Autodesk Inventor part; units mm, degrees
ref_plane "YZ Plane" through (0, 0, 0) normal (1, 0, 0) x (0, 1, 0)
ref_plane "XZ Plane" through (0, 0, 0) normal (0, 1, 0) x (-1, 0, 0)
ref_plane "XY Plane" through (0, 0, 0) normal (0, 0, 1) x (1, 0, 0)
ref_plane "Arbeitsebene1" through (107, -8, 0) normal (-1, 0, 0) x (0, 0, 1)
sketch "Skizze1" plane through (107, -8, 0) normal (-1, 0, 0) x (0, 0, 1)
  line L0 (-4.1, -2) -> (-4.1, -37.1)
  line L1 (0, -2) -> (-4.1, -2)
  line L2 (0, -37.1) -> (0, -2)
  line L3 (0, -37.1) -> (-4.1, -37.1)
  line L4 (0, -37.1) -> (10.7454, -47.8454)
  line L5 (0, -37.1) -> (15.1963, -37.1) construction
  line L6 (10.7454, -47.8454) -> (10.7454, -97.8454)
  line L7 (10.7454, -97.8454) -> (-49.2546, -97.8454)
  line L8 (-49.2546, -97.8454) -> (-49.2546, -102.8454)
  line L9 (-49.2546, -102.8454) -> (15.7454, -102.8454)
  line L10 (15.7454, -102.8454) -> (15.7454, -45.7743)
  line L11 (15.7454, -45.7743) -> (5, -35.0289)
  line L12 (5, -35.0289) -> (5, -2)
  line L13 (5, -2) -> (0, -2)
  line L14 (0, -37.1) -> (0, -2)
  point P0 (0, 8)
  dimension "d0" = 45
  dimension "d1" = 5
  dimension "d2" = 5
  dimension "d3" = 5
  dimension "d4" = 5
  dimension "d5" = 60
  dimension "d6" = 50
extrude "Extrusion1" add sketch "Skizze1" against normal blind 5 contours L13 L12 L11 L10 L9 L8 L7 L6 L4 L2
sketch "Skizze2" plane through (107, -43.0289, 5) normal (0, 0, 1) x (1, 0, 0)
  line L0 (0, 0) -> (0, 33.0289)
  line L1 (0, 0) -> (5, 0)
  line L2 (5, 33.0289) -> (5, 0)
  line L3 (0, 33.0289) -> (5, 33.0289)
  circle A0 centre (2.5, 27.9533) radius 0.9
  circle A1 centre (2.5, 6.9011) radius 0.9
  point P0 (-107, 43.0289)
  dimension "d9" = 1.8
  dimension "d10" = 1.8
extrude "Extrusion2" cut sketch "Skizze2" against normal through all contours A0 | A1
chamfer "Fase1" distance 5 angle 45 2 edges at (109.5, -110.8454, 15.7454) (109.5, -105.8454, 10.7454)
properties part number "07_Omnivision_Lamp_arm"
Design review of the part built by this model. Coordinates are the model's own, in mm. A direction names the side the tool comes from. Coordinates: 2 decimals unless noted, no trailing zeros. Order: outer loops, then holes, each group sorted by start corner. A loop starts at its lowest first (then second) coordinate and runs counter-clockwise, first axis right, second up.
Item 1: The part is to be moulded in two halves that separate along Y. For faces 4 (the flat face through (109, -27, 5)), 5 (the flat face through (109, -78, 10.745)), 6 (the flat face through (109.5, -50.4, 5.3)), 7 (the flat face through (109.54, -108.38, 13.21)), say which applies: pulls with the +Y half, pulls with the -Y half, needs draft (parallel to the pull), parting line crosses it, or undercut.
Item 2: Take a section at B-B, the plane y = -24. Write out the cut boundary in (x, z).
Item 3: For line 1 (Y direction, x = 108.7, z = 1.5); line 2 (Y direction, x = 109.5, z = 3.35); line 3 (Y direction, x = 108.85, z = -38), list the stretches that pass through material, from the lowest coordinate up.
Item 4: Take a section at A-A, the plane x = 109.5. Write out the cut boundary in (y, z), then the cut area to 3 significant figures.
Item 5: For pin 1 Ø2 at (x, y) = (111.5, -39) entering from -Z; pin 2 Ø2.5 at (x, z) = (109.5, -12) entering from +Y; pin 3 Ø1.4 at (x, y) = (109.5, -36.13) entering from -Z; pin 4 Ø1.5 at (x, y) = (108.5, -25.5) entering from +Z, all flat-tipped, find the tip position at first contact; note any pin that passes through.
Item 6: Take a section at C-C, the plane z = -2. Write out the cut boundary in (x, y), then the cut area to 3 significant figures.
Item 7: For faces 1 (the flat face through (109.46, -103.31, 8.28)), 2 (the flat face through (109, -28, 0)), 3 (the flat face through (109.46, -48.48, 10.45)), list the 3-axis set-ups (+Z, -Z, +X, -X, +Y, -Y) from which the entire face can be reached by the end or side of a thin tool; tool diameter is ignored.
The answers:
1. face 4: needs draft
1. face 5: undercut
1. face 6: undercut
1. face 7: pulls with the -Y half
2. outline: (107, 0) - (112, 0) - (112, 5) - (107, 5) - close
3. line 1: y = -110.85 to -105.85, -46.6 to -36.54, -35.72 to -15.49, -14.66 to -10
3. line 2: y = -110.85 to -105.85, -48.45 to -37.03, -35.23 to -15.98, -14.18 to -10
3. line 3: y = -110.85 to -105.85
4. outline: (-110.85, -49.25) - (-105.85, -49.25) - (-105.85, 5.75) - (-100.85, 10.75) - (-55.85, 10.75) - (-45.1, 0) - (-37.03, 0) - (-37.03, 5) - (-43.03, 5) - (-53.77, 15.75) - (-105.85, 15.75) - (-110.85, 10.75) - close; (-35.23, 0) - (-15.98, 0) - (-15.98, 5) - (-35.23, 5) - close; (-14.18, 0) - (-10, 0) - (-10, 5) - (-14.18, 5) - close
4. area: 808 mm2
5. pin 1: stops at z = 0
5. pin 2: stops at y = -105.85
5. pin 3: passes through
5. pin 4: stops at z = 5
6. outline: (107, -110.85) - (112, -110.85) - (112, -105.85) - (107, -105.85) - close
6. area: 25.0 mm2
7. face 1: -Z, +X, -X
7. face 2: -Z, +X, -X, +Y
7. face 3: +Z, +X, -X, +Y
